```python
from build123d import *

# Parameters (mm, degrees)
SKETCH_2_W          = 15
SKETCH_2_H          = 6
SKETCH_2_W_2        = 13.8
SKETCH_2_H_2        = 4.8
EXTRUDE_1_DEPTH     = 50
SKETCH_3_R          = 1.5
CUT_EXTRUDE_1_DEPTH = 80


with BuildPart() as part:
    # 草图2 → 凸台-拉伸1 (new body)
    with BuildSketch(Plane.XY):
        Rectangle(SKETCH_2_W, SKETCH_2_H)
        Rectangle(SKETCH_2_W_2, SKETCH_2_H_2, mode=Mode.SUBTRACT)
    extrude(amount=EXTRUDE_1_DEPTH)

    # 草图3 → 切除-拉伸1 (cut)
    with BuildSketch(Plane(origin=(0, 3, 0), x_dir=(1, 0, 0), z_dir=(0, 1, 0))):
        with Locations(Location((-4, -4, 0), (0, 0, 270))):
            Circle(SKETCH_3_R)
        with Locations(Location((4, -4, 0), (0, 0, 270))):
            Circle(SKETCH_3_R)
        with Locations((4, -46)):
            Circle(SKETCH_3_R)
        with Locations((-4, -46)):
            Circle(SKETCH_3_R)
    extrude(amount=-CUT_EXTRUDE_1_DEPTH, mode=Mode.SUBTRACT)


solid = part.part
```
Could you check a few things on this model? Use its own coordinates, in mm. A direction names the side the tool comes from. Give positions to 0.01 mm unless a question says otherwise; leave off trailing zeros. Write each loop counter-clockwise with the first axis right and the second up, starting at its lowest first coordinate (ties: lowest second). Pieces come first, ordered by that corner, then holes. Notation, with made-up numbers: (56, -17) -> (64, -17) arc R25 ccw to (64, -3) -> close; hole circle Ø9 at (-33.75, 73). An arc over 180 degrees is marked (long way). Write each question's results on one line, items separated by ' | '.
1. On a 3-axis mill with a long thin cutter (end or side, diameter ignored), from which of +Z, -Z, +X, -X, +Y, -Y can I reach the whole of each face in a straight line? I mean faces 4 (the flat face through (6.9, 0, 25)), 5 (the cylindrical face through (-4.325, -2.696, 47.464)). Say none if no direction works.
Check sheet entries:
face 4: +Z, -Z | face 5: +Y, -Y
2. I want a section at D-D, the plane x = 4. Write out the boundary of the cut face in (y, z), then the cut area to 3 significant figures.
Check sheet entries:
outline: (-3, 0) -> (-2.4, 0) -> (-2.4, 2.5) -> (-3, 2.5) -> close; (-3, 5.5) -> (-2.4, 5.5) -> (-2.4, 44.5) -> (-3, 44.5) -> close; (-3, 47.5) -> (-2.4, 47.5) -> (-2.4, 50) -> (-3, 50) -> close; (2.4, 0) -> (3, 0) -> (3, 2.5) -> (2.4, 2.5) -> close; (2.4, 5.5) -> (3, 5.5) -> (3, 44.5) -> (2.4, 44.5) -> close; (2.4, 47.5) -> (3, 47.5) -> (3, 50) -> (2.4, 50) -> close | area: 52.8 mm²
3. I want a section at C-C, the plane z = 4. Write out the boundary of the cut face in (x, y), then the cut area to 3 significant figures.
Check sheet entries:
outline: (-7.5, -3) -> (-5.5, -3) -> (-5.5, -2.4) -> (-6.9, -2.4) -> (-6.9, 2.4) -> (-5.5, 2.4) -> (-5.5, 3) -> (-7.5, 3) -> close; (-2.5, -3) -> (2.5, -3) -> (2.5, -2.4) -> (-2.5, -2.4) -> close; (-2.5, 2.4) -> (2.5, 2.4) -> (2.5, 3) -> (-2.5, 3) -> close; (5.5, -3) -> (7.5, -3) -> (7.5, 3) -> (5.5, 3) -> (5.5, 2.4) -> (6.9, 2.4) -> (6.9, -2.4) -> (5.5, -2.4) -> close | area: 16.6 mm²
4. If we mould it in two halves opening along X, with no side actions, what happens to faces 1 (the flat face through (0, -2.7, 0)), 2 (the flat face through (7.5, 0, 25)), 3 (the flat face through (-6.9, 0, 25))? For each: released by +X, released by -X, zero draft, split by the parting line, or undercut.
Check sheet entries:
face 1: zero draft | face 2: released by +X | face 3: undercut
5. I need wall thicknesses on L1, parallel to X at y = -2.55, z = 4; L2, parallel to Y at x = -5.75, z = 4; L3, parallel to X at y = -0.65, z = 9. Which ranges of each line are inside material? Lowest first, please.
Check sheet entries:
L1: x = -7.5 to -5.5, -2.5 to 2.5, 5.5 to 7.5 | L2: y = -3 to -2.4, 2.4 to 3 | L3: x = -7.5 to -6.9, 6.9 to 7.5
6. I want a section at A-A, the plane x = 1. Write out the boundary of the cut face in (y, z), then the cut area to 3 significant figures.
Check sheet entries:
outline: (-3, 0) -> (-2.4, 0) -> (-2.4, 50) -> (-3, 50) -> close; (2.4, 0) -> (3, 0) -> (3, 50) -> (2.4, 50) -> close | area: 60.0 mm²
7. I want a section at B-B, the plane y = 1.05. Write out the boundary of the cut face in (x, z), then the cut area to 3 significant figures.
Check sheet entries:
outline: (-7.5, 0) -> (-6.9, 0) -> (-6.9, 50) -> (-7.5, 50) -> close; (6.9, 0) -> (7.5, 0) -> (7.5, 50) -> (6.9, 50) -> close | area: 60.0 mm²
